Can you work these out from the model? Positions are in its coordinate system, mm. Face numbers are marked on the shaded views. A direction names the side the tool comes from. Round coordinates to 2 decimals unless told otherwise and drop trailing zeros. Loops run counter-clockwise (first coordinate to the right, second up) from the corner with the lowest first, then second, coordinate; pieces in that order, holes last. Notation, with made-up numbers: (-2, 85) -> (57, 85) arc R13 cw to (57, 103) -> close; hole circle Ø5 at (-12.75, 9.5). An arc over 180 degrees is marked (long way). Answer as a JSON object with one key per item and string values.
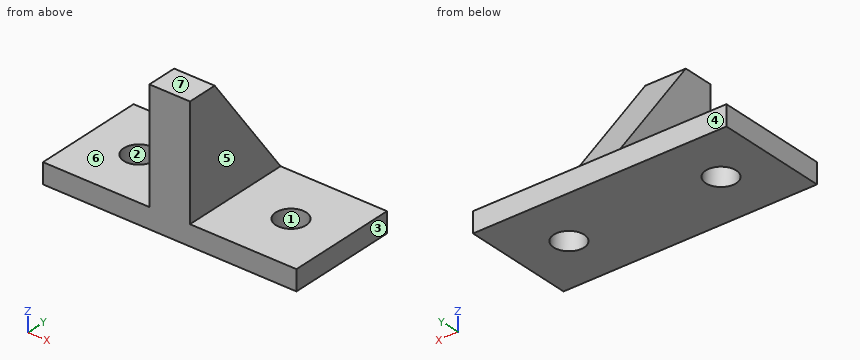
```python
from build123d import *

# Parameters (mm, degrees)
SKETCH1_W                = 125
SKETCH1_H                = 55
SKETCH1_R                = 7.5
BOSS_EXTRUDE1_DEPTH      = 10
BOSS_EXTRUDE2_DEPTH      = 10
BOSS_EXTRUDE2_DEPTH_BACK = 10


with BuildPart() as part:
    # Sketch1 → Boss-Extrude1 (new body)
    with BuildSketch(Plane.XY):
        Rectangle(SKETCH1_W, SKETCH1_H)
        with Locations((37.5, 0)):
            Circle(SKETCH1_R, mode=Mode.SUBTRACT)
        with Locations(Location((-37.5, 0, 0), (0, 0, 180))):
            Circle(SKETCH1_R, mode=Mode.SUBTRACT)
    extrude(amount=BOSS_EXTRUDE1_DEPTH)

    # Sketch2 → Boss-Extrude2 (add, two sides: drawn at the far end of the back side and taken through both)
    with BuildSketch(Plane(origin=(0, 0, 0), x_dir=(0, 0, -1), z_dir=(1, 0, 0)).offset(-BOSS_EXTRUDE2_DEPTH_BACK)):
        Polygon((-10, -27.5), (-65, -27.5), (-65, -12.5), (-10, 27.5), align=None)
    extrude(amount=BOSS_EXTRUDE2_DEPTH + BOSS_EXTRUDE2_DEPTH_BACK)


solid = part.part
```
Q1. If I drill on L1, parallel to Y at x = -37.5, z = 3; L2, parallel to Z at x = -12.5, y = 24; L3, parallel to X at y = -16.5, z = 18.5, over which ranges is the centre line in solid material (lowest first)? Write a range as [from, to].
Determined:
{"L1": "[-27.5, -7.5], [7.5, 27.5]", "L2": "[0, 10]", "L3": "[-10, 10]"}
Q2. I'm going to push flat-ended pins straight in: pin 1 (2 mm diameter, centred on y = -18, z = 41, fed in from +X); pin 2 (1 mm diameter, centred on y = -10.5, z = 46, fed in from -X); pin 3 (13.5 mm diameter, centred on x = -37.5, y = 0, fed in from -Z); pin 4 (2 mm diameter, centred on x = 43.5, y = 6, fed in from +Z). Where does each tip first touch, or does it pass through?
Determined:
{"pin 1": "x = 10", "pin 2": "x = -10", "pin 3": "through", "pin 4": "z = 10"}
Q3. On a 3-axis mill with a long thin cutter (end or side, diameter ignored), from which of +Z, -Z, +X, -X, +Y, -Y can I reach the whole of each face in a straight line? I mean the marked faces 5, 6 and 7. Say none if no direction works.
Determined:
{"face 5": "+Z, +X, +Y, -Y", "face 6": "+Z, -X, +Y, -Y", "face 7": "+Z, +X, -X, +Y, -Y"}
Q4. We'd pull the mould along Y, two halves only. Please class the marked faces 1, 2, 3 and 4: pulls with the +Y half, pulls with the -Y half, needs draft (parallel to the pull), parting line crosses it, or undercut.
Determined:
{"face 1": "undercut", "face 2": "undercut", "face 3": "needs draft", "face 4": "pulls with the +Y half"}
Q5. I want a section at B-B, the plane y = -19.5. Write out the boundary of the cut face in (x, z), then the cut area to 3 significant figures.
Determined:
{"outline": "(-62.5, 0) -> (62.5, 0) -> (62.5, 10) -> (10, 10) -> (10, 65) -> (-10, 65) -> (-10, 10) -> (-62.5, 10) -> close", "area": "2,350 mm²"}
Q6. I want a section at D-D, the plane x = 4. Write out the boundary of the cut face in (y, z), then the cut area to 4 significant figures.
Determined:
{"outline": "(-27.5, 0) -> (27.5, 0) -> (27.5, 10) -> (-12.5, 65) -> (-27.5, 65) -> close", "area": "2,475 mm²"}
Q7. I want a section at C-C, the plane y = 0. Write out the boundary of the cut face in (x, z), then the cut area to 3 significant figures.
Determined:
{"outline": "(-62.5, 0) -> (-45, 0) -> (-45, 10) -> (-62.5, 10) -> close; (-30, 0) -> (30, 0) -> (30, 10) -> (10, 10) -> (10, 47.81) -> (-10, 47.81) -> (-10, 10) -> (-30, 10) -> close; (45, 0) -> (62.5, 0) -> (62.5, 10) -> (45, 10) -> close", "area": "1,710 mm²"}
Q8. I want a section at A-A, the plane x = -37.5. Write out the boundary of the cut face in (y, z), then the cut area to 3 significant figures.
Determined:
{"outline": "(-27.5, 0) -> (-7.5, 0) -> (-7.5, 10) -> (-27.5, 10) -> close; (7.5, 0) -> (27.5, 0) -> (27.5, 10) -> (7.5, 10) -> close", "area": "400 mm²"}
